Geometry: final body of the model. Coordinates: model frame, mm. A direction names the side the tool comes from. Give positions to 0.01 mm unless a question says otherwise; leave off trailing zeros. Write each loop counter-clockwise with the first axis right and the second up, starting at its lowest first coordinate (ties: lowest second). Pieces come first, ordered by that corner, then holes. Notation, with made-up numbers: (62.5, 37.5) - (105.5, 37.5) arc R10 ccw to (105.5, 50.5) - close; hole circle Ø8 at (52, 46). An arc over 180 degrees is marked (long way). Return JSON: item names as keys, results as strings.
from build123d import *

# Parameters (mm, degrees)
BOSS_EXTRUDE1_DEPTH = 2.9
CUT_EXTRUDE1_DEPTH  = 3.9


with BuildPart() as part:
    # Sketch1 → Boss-Extrude1 (new body)
    with BuildSketch(Plane.XY):
        with BuildLine():
            Line((206.1, -203.2), (236.1, -203.2))
            Line((236.1, -203.2), (236.1, -118.2))
            Line((236.1, -118.2), (233.2, -118.2))
            Line((233.2, -118.2), (233.2, -93.2))
            Line((233.2, -93.2), (236.1, -93.2))
            Line((236.1, -93.2), (236.1, 118.2))
            Line((236.1, 118.2), (233.2, 118.2))
            Line((233.2, 118.2), (233.2, 143.2))
            Line((233.2, 143.2), (236.1, 143.2))
            Line((236.1, 143.2), (236.1, 203.2))
            Line((236.1, 203.2), (-236.1, 203.2))
            Line((-236.1, 203.2), (-236.1, 143.2))
            Line((-236.1, 143.2), (-233.2, 143.2))
            Line((-233.2, 143.2), (-233.2, 118.2))
            Line((-233.2, 118.2), (-236.1, 118.2))
            Line((-236.1, 118.2), (-236.1, -93.2))
            Line((-236.1, -93.2), (-233.2, -93.2))
            Line((-233.2, -93.2), (-233.2, -118.2))
            Line((-233.2, -118.2), (-236.1, -118.2))
            Line((-236.1, -118.2), (-236.1, -203.2))
            Line((-236.1, -203.2), (-206.1, -203.2))
            ThreePointArc((-206.1, -203.2), (-199.028932188, -200.271067812), (-196.1, -193.2))
            Line((-196.1, -193.2), (-196.1, -188.2))
            ThreePointArc((-196.1, -188.2), (-193.171067812, -181.128932188), (-186.1, -178.2))
            Line((-186.1, -178.2), (186.1, -178.2))
            ThreePointArc((186.1, -178.2), (193.171067812, -181.128932188), (196.1, -188.2))
            Line((196.1, -188.2), (196.1, -193.2))
            ThreePointArc((196.1, -193.2), (199.028932188, -200.271067812), (206.1, -203.2))
        make_face()
    extrude(amount=BOSS_EXTRUDE1_DEPTH)

    # Sketch2 → Cut-Extrude1 (cut, through all)
    with BuildSketch(Plane.XY.offset(2.9)):
        with BuildLine():
            Line((-181.1, 163.2), (181.1, 163.2))
            ThreePointArc((181.1, 163.2), (184.635533906, 161.735533906), (186.1, 158.2))
            Line((186.1, 158.2), (186.1, -133.2))
            ThreePointArc((186.1, -133.2), (184.635533906, -136.735533906), (181.1, -138.2))
            Line((181.1, -138.2), (-181.1, -138.2))
            ThreePointArc((-181.1, -138.2), (-184.635533906, -136.735533906), (-186.1, -133.2))
            Line((-186.1, -133.2), (-186.1, 158.2))
            ThreePointArc((-186.1, 158.2), (-184.635533906, 161.735533906), (-181.1, 163.2))
        make_face()
    extrude(amount=-CUT_EXTRUDE1_DEPTH, mode=Mode.SUBTRACT)


solid = part.part
Q1. Section query A-A, the plane y = 124. Return the cut outline in (x, z).
Answer key:
{"outline": "(-233.2, 0) - (-186.1, 0) - (-186.1, 2.9) - (-233.2, 2.9) - close; (186.1, 0) - (233.2, 0) - (233.2, 2.9) - (186.1, 2.9) - close"}
Q2. Material intervals for probe 1 along Y at (x, z) = (38, 1.35); probe 2 along X at (y, z) = (155.5, 0.9); probe 3 along X at (y, z) = (-118, 2), sorted ascending. Write a range as [from, to].
Answer key:
{"probe 1": "y = [-178.2, -138.2], [163.2, 203.2]", "probe 2": "x = [-236.1, -186.1], [186.1, 236.1]", "probe 3": "x = [-233.2, -186.1], [186.1, 233.2]"}
Q3. Mould query, pull axis X, two halves, no side actions, for faces 1 (the cylindrical face through (198.95, -200.19, 1.43)), 2 (the flat face through (-3, -178, 0)). Classes: pulls with the +X half, pulls with the -X half, needs draft (parallel to the pull), parting line crosses it, or undercut.
Answer key:
{"face 1": "undercut", "face 2": "needs draft"}
Q4. Set-up query: faces 3 (the cylindrical face through (-199.11, -200.35, 1.43)), 4 (the flat face through (-3, -178, 2.9)). Return all of +Z, -Z, +X, -X, +Y, -Y with unobstructed straight access to the full face (end or side cutting, diameter ignored); none if empty.
Answer key:
{"face 3": "+Z, -Z, -Y", "face 4": "+Z, +X, -X, +Y, -Y"}
Q5. Section query B-B, the plane x = 111.5. Return the cut outline in (y, z).
Answer key:
{"outline": "(-178.2, 0) - (-138.2, 0) - (-138.2, 2.9) - (-178.2, 2.9) - close; (163.2, 0) - (203.2, 0) - (203.2, 2.9) - (163.2, 2.9) - close"}
Q6. Pin query (flat end, axial travel): P1, Ø0.9, axis at y = -101, z = 1.5, coming from the -X side; P2, Ø0.9, axis at x = -58, z = 1.5, coming from the -Y side; P3, Ø1.4, axis at y = 137, z = 1, coming from the +X side. Return the tip coordinate at first contact, or that it passes through.
Answer key:
{"P1": "stops at x = -233.2", "P2": "stops at y = -178.2", "P3": "stops at x = 233.2"}
